Part model, mm, in its own coordinate system. Face numbers are marked on the shaded views. A direction names the side the tool comes from. Give positions to 0.01 mm unless a question says otherwise; leave off trailing zeros. Loops run counter-clockwise (first coordinate to the right, second up) from the corner with the lowest first, then second, coordinate; pieces in that order, holes last. Notation, with made-up numbers: M 38,-8 L 88,-8 A31 cw 88,24 Z; hole C -29.5,-35.5 d11. An arc over 180 degrees is marked long. Answer in a Markdown table with one row per item.
from build123d import *

# Parameters (mm, degrees)
F1_DEPTH = 9
F2_W     = 10
F2_H     = 3
F2_W_2   = 6
F3_DEPTH = 11.5
F5_DEPTH = 3


with BuildPart() as f1:
    # F0 (on Front) → F1 (new body)
    with BuildSketch(Plane.XZ):
        Polygon((-1.5, -10), (1.5, -10), (1.5, 10), (-1.5, 10), (-1.5, 5), (-1.5, 0), (-1.5, -5), align=None)
        with BuildLine():
            ThreePointArc((-11.5, 5), (-16.5, 0), (-11.5, -5))
            Line((-11.5, -5), (-11.5, -1.75))
            ThreePointArc((-11.5, -1.75), (-13.25, 0), (-11.5, 1.75))
            Line((-11.5, 1.75), (-11.5, 5))
        make_face()
        with BuildLine():
            Line((-11.5, -5), (-1.5, -5))
            Line((-1.5, -5), (-1.5, 0))
            Line((-1.5, 0), (-1.5, 5))
            Line((-1.5, 5), (-11.5, 5))
            Line((-11.5, 5), (-11.5, 1.75))
            ThreePointArc((-11.5, 1.75), (-10.2625631329, 1.2374368671), (-9.75, 0))
            ThreePointArc((-9.75, 0), (-10.2625631329, -1.2374368671), (-11.5, -1.75))
            Line((-11.5, -1.75), (-11.5, -5))
        make_face()
    extrude(amount=F1_DEPTH)

    # F2 (on face) → F3 (cut)
    with BuildSketch(Plane(origin=(0, 0, -5), x_dir=(1, 0, 0), z_dir=(0, 0, -1))):
        with Locations((-6.5, 4.5)):
            Rectangle(F2_W, F2_H)
        with Locations((-14.5, 4.5)):
            Rectangle(F2_W_2, F2_H)
    extrude(amount=-F3_DEPTH, mode=Mode.SUBTRACT)

    # F4 (on face) → F5 (cut)
    with BuildSketch(Plane(origin=(-1.5, 0, 0), x_dir=(0, -1, 0), z_dir=(-1, 0, 0))):
        with BuildLine():
            ThreePointArc((4.5, -5.5), (3, -7), (4.5, -8.5))
            Line((4.5, -8.5), (4.5, -5.5))
        make_face()
        with BuildLine():
            Line((4.5, -5.5), (4.5, -8.5))
            ThreePointArc((4.5, -8.5), (5.5606601718, -8.0606601718), (6, -7))
            ThreePointArc((6, -7), (5.5606601718, -5.9393398282), (4.5, -5.5))
        make_face()
        with BuildLine():
            ThreePointArc((4.5, 8.5), (3, 7), (4.5, 5.5))
            Line((4.5, 5.5), (4.5, 8.5))
        make_face()
        with BuildLine():
            Line((4.5, 8.5), (4.5, 5.5))
            ThreePointArc((4.5, 5.5), (5.5606601718, 5.9393398282), (6, 7))
            ThreePointArc((6, 7), (5.5606601718, 8.0606601718), (4.5, 8.5))
        make_face()
    extrude(amount=-F5_DEPTH, mode=Mode.SUBTRACT)


solid = f1.part
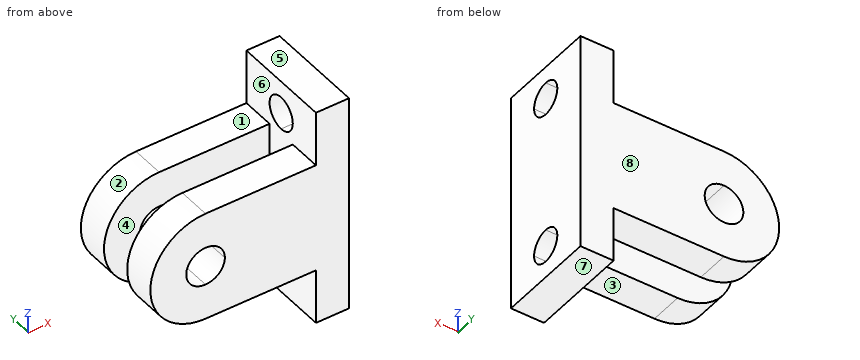
(1) Drill centre lines: line 1 along Y through (x, z) = (-13.75, 3.5); line 2 along Z through (x, y) = (-0.5, -4.25); line 3 along Z through (x, y) = (-0.75, -5). Where is each one in solid material? Low to high.
Recorded:
| item | result |
|---|---|
| line 1 | y = -9 to -6, -3 to 0 |
| line 2 | z = -10 to -8.48, -5.52 to 5.52, 8.48 to 10 |
| line 3 | z = -10 to -8.41, -5.59 to 5.59, 8.41 to 10 |
(2) Saw through at D-D (y = -5.5). Write the cut outline in (x, z), plus the area to 3 significant figures.
Recorded:
| item | result |
|---|---|
| outline | M -1.5,-10 L 1.5,-10 L 1.5,-8.12 L -1.5,-8.12 Z; M -1.5,-5.88 L 1.5,-5.88 L 1.5,5.88 L -1.5,5.88 Z; M -1.5,8.12 L 1.5,8.12 L 1.5,10 L -1.5,10 Z |
| area | 46.6 mm^2 |
(3) Saw through at A-A (x = -0.75). Write the cut outline in (y, z).
Recorded:
| item | result |
|---|---|
| outline | M -9,-10 L 0,-10 L 0,10 L -9,10 Z; hole C -4.5,-7 d3; hole C -4.5,7 d3 |
(4) Pull direction Y, two halves, no side cores. Call the marked faces 6, 7 and 8: +Y half, -Y half, draft (parallel to the pull), parting line (faces both ways), or undercut.
Recorded:
| item | result |
|---|---|
| face 6 | undercut |
| face 7 | draft |
| face 8 | +Y half |
(5) Pin check, flat tips, straight feed: pin 1 Ø2.5 at (y, z) = (-6, 2.5) entering from -X; pin 2 Ø2.5 at (x, y) = (-6.5, -7) entering from -Z; pin 3 Ø2.5 at (x, y) = (-5.5, -8) entering from +Z. Stop position of each tip, or through.
Recorded:
| item | result |
|---|---|
| pin 1 | stops at x = -16.34 |
| pin 2 | stops at z = -5 |
| pin 3 | stops at z = 5 |
(6) Saw through at B-B (y = -2.75). Write the cut outline in (x, z), plus the area to 3 significant figures.
Recorded:
| item | result |
|---|---|
| outline | M -11.5,-5 L -1.5,-5 L -1.5,-10 L 1.5,-10 L 1.5,10 L -1.5,10 L -1.5,5 L -11.5,5 A5 ccw Z; hole C -11.5,0 d3.5 |
| area | 190 mm^2 |
(7) Which spindle directions (+Z, -Z, +X, -X, +Y, -Y) get a long thin tool onto all of the face, cutting with end or side? Do the marked faces 1, 2, 3, 4 and 5. Say none if no direction does.
Recorded:
| item | result |
|---|---|
| face 1 | +Z, -X, +Y, -Y |
| face 2 | -X, +Y, -Y |
| face 3 | -Z, -X, +Y, -Y |
| face 4 | +Z, -Z, -X |
| face 5 | +Z, +X, -X, +Y, -Y |
(8) Saw through at C-C (x = -9). Write the cut outline in (y, z).
Recorded:
| item | result |
|---|---|
| outline | M -9,-5 L -6,-5 L -6,5 L -9,5 Z; M -3,-5 L 0,-5 L 0,5 L -3,5 Z |
